```python
from build123d import *

# Parameters (mm, degrees)
ESQUISSE1_R             = 13
BOSS_EXTRU_1_DEPTH      = 97
ESQUISSE2_R             = 2.5
BOSS_EXTRU_2_DEPTH      = 17
ENL_V_MAT_EXTRU_1_DEPTH = 18.5
ESQUISSE4_R             = 6.5
ESQUISSE4_R_2           = 2.5
BOSS_EXTRU_3_DEPTH      = 2
ESQUISSE5_R             = 1.5
ENL_V_MAT_EXTRU_2_DEPTH = 4
ENL_V_START             = -12
ENL_V_MAT_EXTRU_3_DEPTH = 12


with BuildPart() as part:
    # Esquisse1 → Boss.-Extru.1 (new body)
    with BuildSketch(Plane.XY):
        with Locations(Location((0, 0, 0), (0, 0, 180))):
            Circle(ESQUISSE1_R)
    extrude(amount=BOSS_EXTRU_1_DEPTH)

    # Esquisse2 → Boss.-Extru.2 (add)
    with BuildSketch(Plane.XY.offset(97)):
        Circle(ESQUISSE2_R)
    extrude(amount=BOSS_EXTRU_2_DEPTH)

    # Esquisse3 → Enlèv. mat.-Extru.1 (cut)
    with BuildSketch(Plane(origin=(0, 0, 0), x_dir=(-1, 0, 0), z_dir=(0, 0, -1))):
        with BuildLine():
            Line((-10.5, 0), (-10.5, 4))
            Line((-10.5, 4), (-12.369316877, 4))
            ThreePointArc((-12.369316877, 4), (-13, 0), (-12.369316877, -4))
            Line((-12.369316877, -4), (-10.5, -4))
            Line((-10.5, -4), (-10.5, 0))
        make_face()
        with BuildLine():
            Line((10.5, 0), (10.5, 4))
            Line((10.5, 4), (12.369316877, 4))
            ThreePointArc((12.369316877, 4), (12.99999812, -0.006990598), (12.365007817, -4.013300596))
            Line((12.365007817, -4.013300596), (10.5, -4))
            Line((10.5, -4), (10.5, 0))
        make_face()
    extrude(amount=-ENL_V_MAT_EXTRU_1_DEPTH, mode=Mode.SUBTRACT)

    # Esquisse4 → Boss.-Extru.3 (add)
    with BuildSketch(Plane.XY.offset(97)):
        Circle(ESQUISSE4_R)
        Circle(ESQUISSE4_R_2, mode=Mode.SUBTRACT)
    extrude(amount=BOSS_EXTRU_3_DEPTH)

    # Esquisse5 → Enlèv. mat.-Extru.2 (cut)
    with BuildSketch(Plane.XY.offset(97)):
        with Locations((0, 10)):
            Circle(ESQUISSE5_R)
        with Locations((-10, 0)):
            Circle(ESQUISSE5_R)
        with Locations((0, -10)):
            Circle(ESQUISSE5_R)
        with Locations((10, 0)):
            Circle(ESQUISSE5_R)
    extrude(amount=-ENL_V_MAT_EXTRU_2_DEPTH, mode=Mode.SUBTRACT)

    # Esquisse6 → Enlèv. mat.-Extru.3 (cut)
    with BuildSketch(Plane.XY.offset(114).offset(ENL_V_START)):
        with BuildLine():
            Line((0, 2), (1.5, 2))
            ThreePointArc((1.5, 2), (0, 2.5), (-1.5, 2))
            Line((-1.5, 2), (0, 2))
        make_face()
    extrude(amount=ENL_V_MAT_EXTRU_3_DEPTH, mode=Mode.SUBTRACT)


solid = part.part
```
For this review, take the finished solid that the model builds, in its own axes (mm). A direction names the side the tool comes from. Round coordinates to 2 decimals unless told otherwise and drop trailing zeros. Write each loop counter-clockwise with the first axis right and the second up, starting at its lowest first coordinate (ties: lowest second). Pieces come first, ordered by that corner, then holes. Notation, with made-up numbers: (-5, 61) -> (33, 61) arc R28 cw to (33, 86) -> close; hole circle Ø1 at (15.5, 0). An arc over 180 degrees is marked (long way). Use one line per item in the form item = value.
Q1. Consider section B-B (x = 0). State the section outline as (y, z) points.
Resolved:
outline = (-13, 0) -> (13, 0) -> (13, 97) -> (11.5, 97) -> (11.5, 93) -> (8.5, 93) -> (8.5, 97) -> (6.5, 97) -> (6.5, 99) -> (2.5, 99) -> (2.5, 102) -> (2, 102) -> (2, 114) -> (-2.5, 114) -> (-2.5, 99) -> (-6.5, 99) -> (-6.5, 97) -> (-8.5, 97) -> (-8.5, 93) -> (-11.5, 93) -> (-11.5, 97) -> (-13, 97) -> close
Q2. Consider section A-A (y = 0). State the section outline as (x, z) points.
Resolved:
outline = (-13, 18.5) -> (-10.5, 18.5) -> (-10.5, 0) -> (10.5, 0) -> (10.5, 18.5) -> (13, 18.5) -> (13, 97) -> (11.5, 97) -> (11.5, 93) -> (8.5, 93) -> (8.5, 97) -> (6.5, 97) -> (6.5, 99) -> (2.5, 99) -> (2.5, 114) -> (-2.5, 114) -> (-2.5, 99) -> (-6.5, 99) -> (-6.5, 97) -> (-8.5, 97) -> (-8.5, 93) -> (-11.5, 93) -> (-11.5, 97) -> (-13, 97) -> close
Q3. The part is to be moulded in two halves that separate along Y. For faces 1 (the cylindrical face through (-0.54, -2.44, 106.4)), 2 (the flat face through (0, 10, 93)), 3 (the flat face through (0, 0, 0)), 4 (the flat face through (-12, 0, 18.5)), say which applies: released by +Y, released by -Y, zero draft, split by the parting line, or undercut.
Resolved:
face_1 = split by the parting line
face_2 = undercut
face_3 = zero draft
face_4 = undercut
Q4. Consider section C-C (z = 8). State the section outline as (x, y) points (3 decimals), then the cut area to 3 significant figures.
Resolved:
outline = (-12.369, 4) -> (-10.5, 4) -> (-10.5, -4) -> (-12.365, -4.013) arc R13 ccw to (12.369, -4) -> (10.5, -4) -> (10.5, 4) -> (12.369, 4) arc R13 ccw to start
area = 494 mm²
Q5. Machinability: for faces 5 (the flat face through (-10.5, 0, 9)), 6 (the cylindrical face through (-0.325, 8.536, 95.028)), 7 (the flat face through (10.5, 0, 9)), which of the approach directions +Z, -Z, +X, -X, +Y, -Y give a long, thin tool a straight path to every point of the face, cutting with its end or side? Answer none if there is none.
Resolved:
face_5 = -Z, -X
face_6 = +Z
face_7 = -Z, +X
Q6. Consider section D-D (x = -5). State the section outline as (y, z) points.
Resolved:
outline = (-12, 0) -> (12, 0) -> (12, 97) -> (4.15, 97) -> (4.15, 99) -> (-4.15, 99) -> (-4.15, 97) -> (-12, 97) -> close
Q7. To check wall thickness, follow probe 1 along Y at (x, z) = (0, 95.95); probe 2 along Z at (x, y) = (-5.75, -0.75); probe 3 along Z at (x, y) = (5.5, -5.75). State the ranges of each line that lie inside material, in increasing order. Write a range as from..to.
Resolved:
probe_1 = -13..-11.5, -8.5..8.5, 11.5..13
probe_2 = 0..99
probe_3 = 0..97
Q8. Clearance check with flat-ended pins moving along their axes: pin 1 Ø2.5 at (x, z) = (-0.5, 105.5) entering from +Y; pin 2 Ø0.6 at (x, z) = (11, 14) entering from +Y; pin 3 Ø4 at (x, y) = (0, -10) entering from +Z; pin 4 Ø1.8 at (x, y) = (0, 10) entering from -Z. State where each tip first meets the part, or that it passes through.
Resolved:
pin_1 = 2
pin_2 = 7.38
pin_3 = 97
pin_4 = 0
